```python
from build123d import *

# Parameters (mm, degrees)
EXTRUDE_329_DEPTH = 11


with BuildPart() as part:
    # 草图1 → Extrude 329 (new, symmetric)
    with BuildSketch(Plane.XY):
        Polygon((1.633901262, 2.83), (-1.633901262, 2.83), (-3.267802524, 0), (-1.633901262, -2.83), (1.633901262, -2.83), (3.267802524, 0), align=None)
    extrude(amount=EXTRUDE_329_DEPTH, both=True)

    # 草图3 → 螺纹孔1 (revolve, cut)
    with BuildSketch(Plane(origin=(0, 0, 11), x_dir=(0, -1, 0), z_dir=(1, 0, 0))):
        Polygon((0, 0), (0, 13.951075774), (1.25, 13.2), (1.25, 0), align=None)
    hole_wizard_1 = revolve(axis=Axis((0, 0, 17.35), (0, 0, -1)), mode=Mode.SUBTRACT)

    # 镜向1: 螺纹孔1 across plane
    add(hole_wizard_1.mirror(Plane.XY), mode=Mode.SUBTRACT)


solid = part.part
```
The listing builds one solid part. Answer for the finished solid, in the listing's coordinates (mm). Give positions to 0.01 mm unless a question says otherwise; leave off trailing zeros. Order: outer loops, then holes, each group sorted by start corner. A loop starts at its lowest first (then second) coordinate and runs counter-clockwise, first axis right, second up. Notation, with made-up numbers: (29, 45.25) -> (34, 45.25) arc R23 ccw to (34, 73.25) -> close; hole circle Ø4 at (-17, 69). An arc over 180 degrees is marked (long way). One line per item, written item: value.
1) Find section A-A, the plane z = -4.75. Determine the outline of the cut face in (x, y), plus the area to 3 significant figures.
Reported:
outline: (-3.27, 0) -> (-1.63, -2.83) -> (1.63, -2.83) -> (3.27, 0) -> (1.63, 2.83) -> (-1.63, 2.83) -> close; hole circle Ø2.5 at (0, 0)
area: 22.8 mm^2
2) Find section D-D, the plane y = -1.7. Determine the outline of the cut face in (x, z), plus the area to 3 significant figures.
Reported:
outline: (-2.29, -11) -> (2.29, -11) -> (2.29, 11) -> (-2.29, 11) -> close
area: 101 mm^2
3) Flat-ended cylindrical pins translate along their axes: P1, Ø1.5, axis at y = 1, z = 4, coming from the -X side; P2, Ø1.5, axis at x = -2, z = 2.5, coming from the +Y side; P3, Ø3, axis at y = 2, z = -8, coming from the +X side. Find the tip coordinate at first contact, or state that the pin passes through.
Reported:
P1: stops at x = -3.12
P2: stops at y = 2.83
P3: stops at x = 2.98
4) Find the intervals of material crossed by line 1 (Y direction, x = 0, z = 2.25); line 2 (X direction, y = -0.5, z = -6.5); line 3 (X direction, y = -1.05, z = -8.5), in increasing order.
Reported:
line 1: y = -2.83 to -1.25, 1.25 to 2.83
line 2: x = -2.98 to -1.15, 1.15 to 2.98
line 3: x = -2.66 to -0.68, 0.68 to 2.66
5) Find section C-C, the plane y = 0.45. Determine the outline of the cut face in (x, z), plus the area to 3 significant figures.
Reported:
outline: (-3.01, -11) -> (-1.17, -11) -> (-1.17, 11) -> (-3.01, 11) -> close; (1.17, -11) -> (3.01, -11) -> (3.01, 11) -> (1.17, 11) -> close
area: 81.0 mm^2
6) Find section B-B, the plane x = 0. Determine the outline of the cut face in (y, z), plus the area to 3 significant figures.
Reported:
outline: (-2.83, -11) -> (-1.25, -11) -> (-1.25, 11) -> (-2.83, 11) -> close; (1.25, -11) -> (2.83, -11) -> (2.83, 11) -> (1.25, 11) -> close
area: 69.5 mm^2
7) Determine the mould class of faces 1 (the flat face through (2.46, 1.4, 0.15)), 2 (the flat face through (-2.46, -1.4, 0.15)), 3 (the cylindrical face through (1.22, 0.27, -0.15)) for opening direction X: pulls with the +X half, pulls with the -X half, needs draft (parallel to the pull), parting line crosses it, or undercut.
Reported:
face 1: pulls with the +X half
face 2: pulls with the -X half
face 3: undercut
